from build123d import *

# Parameters (mm, degrees)
F0_W     = 35
F0_H     = 35
F1_DEPTH = 10
F2_SIZE  = 3
F3_R     = 1
F4_R     = 1.5
F5_DEPTH = 10.001
F6_R     = 4.5
F7_DEPTH = 10.001
F9_DEPTH = 4


with BuildPart() as f1:
    # F0 (on Front) → F1 (new body)
    with BuildSketch(Plane.XZ):
        Rectangle(F0_W, F0_H)
    extrude(amount=F1_DEPTH)

    # F2
    f2_edges = [f1.edges().sort_by_distance(p)[0] for p in [
        (-17.5, -5, 17.5),
        (17.5, -5, 17.5),
        (17.5, -5, -17.5),
        (-17.5, -5, -17.5),
    ]]
    chamfer(f2_edges, length=F2_SIZE)

    # F3
    f3_edges = [f1.edges().sort_by_distance(p)[0] for p in [
        (-14.5, -5, 17.5),
        (14.5, -5, 17.5),
        (17.5, -5, 14.5),
        (17.5, -5, -14.5),
        (14.5, -5, -17.5),
        (-14.5, -5, -17.5),
        (-17.5, -5, -14.5),
        (-17.5, -5, 14.5),
    ]]
    fillet(f3_edges, radius=F3_R)

    # F4 (on face) → F5 (cut, through all)
    with BuildSketch(Plane.XZ.offset(10)):
        with Locations((-13, 13)):
            Circle(F4_R)
        with Locations((-13, -13)):
            Circle(F4_R)
        with Locations((13, -13)):
            Circle(F4_R)
        with Locations((13, 13)):
            Circle(F4_R)
    extrude(amount=-F5_DEPTH, mode=Mode.SUBTRACT)

    # F6 (on face) → F7 (cut, through all)
    with BuildSketch(Plane.XZ.offset(10)):
        Circle(F6_R)
    extrude(amount=-F7_DEPTH, mode=Mode.SUBTRACT)

    # F8 (on face) → F9 (cut)
    with BuildSketch(Plane(origin=(0, 0, 0), x_dir=(-1, 0, 0), z_dir=(0, 1, 0))):
        Polygon((12, 17.5), (-12, 17.5), (-17.5, 12), (-17.5, -12), (-12, -17.5), (12, -17.5), (17.5, -12), (17.5, 12), align=None)
    extrude(amount=-F9_DEPTH, mode=Mode.SUBTRACT)


solid = f1.part
Check sheet for the modelled part. Datum: model origin and axes. Units: mm. A direction names the side the tool comes from. Round coordinates to 2 decimals unless told otherwise and drop trailing zeros. Loops run counter-clockwise (first coordinate to the right, second up) from the corner with the lowest first, then second, coordinate; pieces in that order, holes last. Notation, with made-up numbers: (-30, 65.5) -> (-15, 65.5) arc R17 ccw to (-15, 96.5) -> close; hole circle Ø6 at (30.25, 78.25). An arc over 180 degrees is marked (long way). Put each result on its own line as item: value. Start each with the question number.
1. Access from +Z, -Z, +X, -X, +Y, -Y to the whole of each face (thin tool, end or side, straight path). Record for faces 4 (the face through (-16, -5, 16)), 5 (the face through (-14.7, -2, -14.8)).
2. Section check B-B (x = 13). Enter the section's corners in (y, z), plus the area to 3 significant figures.
3. Section check C-C (z = 13). Enter the section's corners in (x, y), plus the area to 3 significant figures.
4. Section check D-D (x = 0). Enter the section's corners in (y, z), plus the area to 3 significant figures.
5. Gauge pin test, flat ends, axial feed: pin 1 (14.5 mm diameter, centred on x = 0, z = 0, fed in from -Y); pin 2 (12 mm diameter, centred on x = -7, z = -6.5, fed in from +Y). Record the tip position at first contact, or that the pin passes through.
6. Draft check along X on faces 1 (the face through (-17.5, -6, 0)), 2 (the face through (14.8, -2, -14.7)), 3 (the face through (16, -5, -16)). Enter one of: +X half, -X half, draft (parallel to the pull), parting line (faces both ways), or undercut.
7. Section check A-A (y = -3.5). Enter the section's corners in (x, z).
8. Scan lines: probe 1 along Z at (x, y) = (13, -5.7); probe 2 along Z at (x, y) = (0, -8.6); probe 3 along Y at (x, z) = (-13, 0.5). Record each from-to range of solid material in increasing order.
Findings:
1. face 4: +Z, -X, +Y, -Y
1. face 5: +Y
2. outline: (-10, -17.5) -> (0, -17.5) -> (0, -16.5) -> (-4, -16.5) -> (-4, -14.5) -> (-10, -14.5) -> close; (-10, -11.5) -> (-4, -11.5) -> (-4, 11.5) -> (-10, 11.5) -> close; (-10, 14.5) -> (-4, 14.5) -> (-4, 16.5) -> (0, 16.5) -> (0, 17.5) -> (-10, 17.5) -> close
2. area: 182 mm^2
3. outline: (-17.5, -10) -> (-14.5, -10) -> (-14.5, -4) -> (-16.5, -4) -> (-16.5, 0) -> (-17.5, 0) -> close; (-11.5, -10) -> (11.5, -10) -> (11.5, -4) -> (-11.5, -4) -> close; (14.5, -10) -> (17.5, -10) -> (17.5, 0) -> (16.5, 0) -> (16.5, -4) -> (14.5, -4) -> close
3. area: 182 mm^2
4. outline: (-10, -17.5) -> (-4, -17.5) -> (-4, -4.5) -> (-10, -4.5) -> close; (-10, 4.5) -> (-4, 4.5) -> (-4, 17.5) -> (-10, 17.5) -> close
4. area: 156 mm^2
5. pin 1: stops at y = -10
5. pin 2: stops at y = -4
6. face 1: -X half
6. face 2: undercut
6. face 3: +X half
7. outline: (-17.5, -14.09) arc R1 ccw to (-17.21, -14.79) -> (-14.79, -17.21) arc R1 ccw to (-14.09, -17.5) -> (-12, -17.5) -> (-17.5, -12) -> close; (-17.5, 12) -> (-12, 17.5) -> (-14.09, 17.5) arc R1 ccw to (-14.79, 17.21) -> (-17.21, 14.79) arc R1 ccw to (-17.5, 14.09) -> close; (12, -17.5) -> (14.09, -17.5) arc R1 ccw to (14.79, -17.21) -> (17.21, -14.79) arc R1 ccw to (17.5, -14.09) -> (17.5, -12) -> close; (12, 17.5) -> (17.5, 12) -> (17.5, 14.09) arc R1 ccw to (17.21, 14.79) -> (14.79, 17.21) arc R1 ccw to (14.09, 17.5) -> close
8. probe 1: z = -17.5 to -14.5, -11.5 to 11.5, 14.5 to 17.5
8. probe 2: z = -17.5 to -4.5, 4.5 to 17.5
8. probe 3: y = -10 to -4
